Build history of the part. All positions in model axes, mm. A direction names the side the tool comes from. Give positions to 0.01 mm unless a question says otherwise; leave off trailing zeros. Write each loop counter-clockwise with the first axis right and the second up, starting at its lowest first coordinate (ties: lowest second). Pieces come first, ordered by that corner, then holes. Notation, with made-up numbers: (51, 7.5) -> (59, 7.5) arc R5 ccw to (59, 16.5) -> close; hole circle Ø4 at (45.25, 67.25). An arc over 180 degrees is marked (long way). Write item = value, one per line. Start each with the question number.
Q1. Saw through at C-C, the plane y = 4. List the corners of the cut face in (x, z) (3 decimals).
Q2. Saw through at A-A, the plane z = 0.95. List the corners of the cut face in (x, y) (3 decimals).
Q3. Tool access for faces 1 (the face through (-0.225, -3, 1)), 2 (the face through (0.225, 0, 1)), 3 (the face through (-0.225, 0, -0.5)): list every direction of +Z, -Z, +X, -X, +Y, -Y with a clear straight run to the whole face (end or side of a thin tool).
Q4. Wall check: line 1 (X direction, y = -3, z = -0.15) (3 decimals); line 2 (Z direction, x = -1.2, y = 0.5); line 3 (Z direction, x = -0.1, y = 2.75). Give the ranges that are in metal, low to high.
Q5. Drop flat-ended pins along their axis: P1, Ø1.5, axis at y = -1.5, z = 1.5, coming from the -X side; P2, Ø1.5, axis at x = -2, y = -3.5, coming from the -Z side; P3, Ø2, axis at x = 1.5, y = 2.5, coming from the +Z side. Give the stop position or say it passes through.
Q6. Saw through at D-D, the plane z = 0.25. List the corners of the cut face in (x, y).
Q7. Saw through at B-B, the plane x = 2.45. List the corners of the cut face in (y, z).
from build123d import *
from OCP.BRepFilletAPI import BRepFilletAPI_MakeChamfer

# Parameters (mm, degrees)
SKETCH_1_W                     = 5.5
SKETCH_1_H                     = 10.5
EXTRUDE_1_DEPTH                = 0.8
SKETCH_2_W                     = 1
SKETCH_2_H                     = 2
CUT_EXTRUDE_1_DEPTH            = 6.980384603
SKETCH_3_W                     = 0.45
SKETCH_3_H                     = 1.5
EXTRUDE_2_DEPTH                = 2.5
SKETCH_5_W                     = 1.8
SKETCH_5_H                     = 0.2
CUT_EXTRUDE_2_DEPTH            = 7.877726732
FILLET_5_R                     = 0.65
CHAMFER_1_SIZE                 = 0.3
CHAMFER_1_SIZE_2               = 0.2
CUT_EXTRUDE_3_DEPTH            = 7.877726732
FILLET_6_R                     = 0.1
PATTERN_LINEAR_1_COUNT         = 3
PATTERN_LINEAR_1_PITCH         = 2.9
FILLET_6_OF_PATTERN_LINEAR_1_R = 0.1
SKETCH_3_2_W                   = 0.45
SKETCH_3_2_H                   = 1.5
EXTRUDE_3_DEPTH                = 1.4
SKETCH_8_W                     = 0.5
SKETCH_8_H                     = 2.5
EXTRUDE_4_DEPTH                = 0.45


with BuildPart() as part:
    # 草图1 → 凸台-拉伸1 (new body)
    with BuildSketch(Plane.XY):
        Rectangle(SKETCH_1_W, SKETCH_1_H)
    extrude(amount=EXTRUDE_1_DEPTH)

    # 草图2 → 切除-拉伸1 (cut, through all)
    with BuildSketch(Plane(origin=(0, 0, 0), x_dir=(-1, 0, 0), z_dir=(0, 0, -1))):
        with Locations((-2.75, 2.75)):
            Rectangle(SKETCH_2_W, SKETCH_2_H)
        with Locations((-2.75, -2.75)):
            Rectangle(SKETCH_2_W, SKETCH_2_H)
        with Locations((2.75, -2.75)):
            Rectangle(SKETCH_2_W, SKETCH_2_H)
        with Locations((2.75, 2.75)):
            Rectangle(SKETCH_2_W, SKETCH_2_H)
    extrude(amount=-CUT_EXTRUDE_1_DEPTH, mode=Mode.SUBTRACT)

    # 草图3 → 凸台-拉伸2 (add)
    with BuildSketch(Plane.XY.offset(0.8)):
        with Locations((0, 2.9)):
            Rectangle(SKETCH_3_W, SKETCH_3_H)
        Rectangle(SKETCH_3_W, SKETCH_3_H)
        with Locations((0, -2.9)):
            Rectangle(SKETCH_3_W, SKETCH_3_H)
    extrude(amount=EXTRUDE_2_DEPTH)

    # 草图5 → 切除-拉伸2 (cut, through all)
    with BuildSketch(Plane.ZY.offset(0.225)):
        with Locations((2.4, 2.25)):
            Rectangle(SKETCH_5_W, SKETCH_5_H)
        with Locations((2.4, -0.65)):
            Rectangle(SKETCH_5_W, SKETCH_5_H)
        with Locations((2.4, -3.55)):
            Rectangle(SKETCH_5_W, SKETCH_5_H)
    extrude(amount=-CUT_EXTRUDE_2_DEPTH, mode=Mode.SUBTRACT)

    # 圆角5
    fillet_5_edges = [part.edges().sort_by_distance(p)[0] for p in [
        (0, -3.45, 3.3),
        (0, -2.15, 3.3),
        (0, -0.55, 3.3),
        (0, 0.75, 3.3),
        (0, 2.35, 3.3),
        (0, 3.65, 3.3),
    ]]
    fillet(fillet_5_edges, radius=FILLET_5_R - 0.0001)  # a hair under: the kernel refuses the full size

    # 倒角1
    chamfer_1_edges_1 = [part.edges().sort_by_distance(p)[0] for p in [
        (0, 2.15, 1.5),
    ]]
    chamfer_1_side_1 = [part.faces().sort_by_distance(p)[0] for p in [
        (0, 2.15, 1.496),
    ]]
    chamfer_1_edges_2 = [part.edges().sort_by_distance(p)[0] for p in [
        (0, -0.75, 1.5),
    ]]
    chamfer_1_side_2 = [part.faces().sort_by_distance(p)[0] for p in [
        (0, -0.75, 1.496),
    ]]
    chamfer_1_edges_3 = [part.edges().sort_by_distance(p)[0] for p in [
        (0, -3.65, 1.5),
    ]]
    chamfer_1_side_3 = [part.faces().sort_by_distance(p)[0] for p in [
        (0, -3.65, 1.496),
    ]]
    chamfer_1 = BRepFilletAPI_MakeChamfer(part.part.solid().wrapped)
    for e in chamfer_1_edges_1:
        chamfer_1.Add(CHAMFER_1_SIZE - 0.0001, CHAMFER_1_SIZE_2 - 0.0001, e.wrapped, chamfer_1_side_1[0].wrapped)
    for e in chamfer_1_edges_2:
        chamfer_1.Add(CHAMFER_1_SIZE - 0.0001, CHAMFER_1_SIZE_2 - 0.0001, e.wrapped, chamfer_1_side_2[0].wrapped)
    for e in chamfer_1_edges_3:
        chamfer_1.Add(CHAMFER_1_SIZE - 0.0001, CHAMFER_1_SIZE_2 - 0.0001, e.wrapped, chamfer_1_side_3[0].wrapped)
    add(Compound.cast(chamfer_1.Shape()), mode=Mode.REPLACE)  # a hair under: the kernel refuses the full size

    # 草图6 → 切除-拉伸3 (cut, through all)
    with BuildSketch(Plane.ZY.offset(0.225)):
        with BuildLine():
            Line((2.7, 2.65), (1.8, 2.65))
            ThreePointArc((1.8, 2.65), (1.647213595, 3.05), (1.8, 3.45))
            Line((1.8, 3.45), (2.7, 3.45))
            ThreePointArc((2.7, 3.45), (2.852786405, 3.05), (2.7, 2.65))
        make_face()
    cut_extrude_3 = extrude(amount=-CUT_EXTRUDE_3_DEPTH, mode=Mode.SUBTRACT)

    # 圆角6
    fillet_6_edges = [part.edges().sort_by_distance(p)[0] for p in [
        (0, 2.65, 1.8),
        (0, 3.45, 1.8),
        (0, 3.45, 2.7),
        (0, 2.65, 2.7),
    ]]
    fillet(fillet_6_edges, radius=FILLET_6_R)

    # 阵列(线性)1: 切除-拉伸3 ×3
    with Locations(*[(0, -i * PATTERN_LINEAR_1_PITCH, 0) for i in range(1, PATTERN_LINEAR_1_COUNT)]):
        add(cut_extrude_3, mode=Mode.SUBTRACT)

    # 圆角6 of 阵列(线性)1
    fillet_6_of_pattern_linear_1_edges = [part.edges().sort_by_distance(p)[0] for p in [
        (0, -0.25, 1.8),
        (0, 0.55, 1.8),
        (0, 0.55, 2.7),
        (0, -0.25, 2.7),
        (0, -3.15, 1.8),
        (0, -2.35, 1.8),
        (0, -2.35, 2.7),
        (0, -3.15, 2.7),
    ]]
    fillet(fillet_6_of_pattern_linear_1_edges, radius=FILLET_6_OF_PATTERN_LINEAR_1_R)

    # 草图3<2> → 凸台-拉伸3 (add)
    with BuildSketch(Plane.XY.offset(0.8)):
        with Locations((0, 2.9)):
            Rectangle(SKETCH_3_2_W, SKETCH_3_2_H)
        Rectangle(SKETCH_3_2_W, SKETCH_3_2_H)
        with Locations((0, -2.9)):
            Rectangle(SKETCH_3_2_W, SKETCH_3_2_H)
    extrude(amount=-EXTRUDE_3_DEPTH)

    # 草图8 → 凸台-拉伸4 (add)
    with BuildSketch(Plane.ZY.offset(0.225)):
        with Locations((-0.35, -2.9)):
            Rectangle(SKETCH_8_W, SKETCH_8_H)
        with Locations((-0.35, 2.9)):
            Rectangle(SKETCH_8_W, SKETCH_8_H)
        with BuildLine():
            Line((-0.6, -1.25), (-0.1, -1.25))
            Line((-0.1, -1.25), (-0.1, 1.25))
            Line((-0.1, 1.25), (-0.6, 1.25))
            ThreePointArc((-0.6, 1.25), (-1.0387505, 0), (-0.6, -1.25))
        make_face()
    extrude(amount=-EXTRUDE_4_DEPTH)


solid = part.part
Report:
q1.outline = (-2.75, 0) -> (2.75, 0) -> (2.75, 0.8) -> (-2.75, 0.8) -> close; (-0.225, -0.6) -> (0.225, -0.6) -> (0.225, -0.1) -> (-0.225, -0.1) -> close
q2.outline = (-0.225, -3.65) -> (0.225, -3.65) -> (0.225, -2.15) -> (-0.225, -2.15) -> close; (-0.225, -0.75) -> (0.225, -0.75) -> (0.225, 0.75) -> (-0.225, 0.75) -> close; (-0.225, 2.15) -> (0.225, 2.15) -> (0.225, 3.65) -> (-0.225, 3.65) -> close
q3.face_1 = +Z, -X, +Y, -Y
q3.face_2 = +Z, +X, +Y, -Y
q3.face_3 = -Z, -X, +Y, -Y
q4.line_1 = -0.225 to 0.225
q4.line_2 = 0 to 0.8
q4.line_3 = -0.6 to 1.73, 2.77 to 3.25
q5.P1 = -2.75
q5.P2 = 0
q5.P3 = 0.8
q6.outline = (-2.75, -5.25) -> (2.75, -5.25) -> (2.75, -3.75) -> (2.25, -3.75) -> (2.25, -1.75) -> (2.75, -1.75) -> (2.75, 1.75) -> (2.25, 1.75) -> (2.25, 3.75) -> (2.75, 3.75) -> (2.75, 5.25) -> (-2.75, 5.25) -> (-2.75, 3.75) -> (-2.25, 3.75) -> (-2.25, 1.75) -> (-2.75, 1.75) -> (-2.75, -1.75) -> (-2.25, -1.75) -> (-2.25, -3.75) -> (-2.75, -3.75) -> close
q7.outline = (-5.25, 0) -> (-3.75, 0) -> (-3.75, 0.8) -> (-5.25, 0.8) -> close; (-1.75, 0) -> (1.75, 0) -> (1.75, 0.8) -> (-1.75, 0.8) -> close; (3.75, 0) -> (5.25, 0) -> (5.25, 0.8) -> (3.75, 0.8) -> close
